```python
from build123d import *

# Parameters (mm, degrees)
SKETCH1_W           = 27.5
SKETCH1_H           = 40
BOSS_EXTRUDE1_DEPTH = 6.5
SKETCH2_W           = 17.25
SKETCH2_H           = 15.4
CUT_EXTRUDE1_DEPTH  = 1.15
SKETCH3_W           = 15.312161922
SKETCH3_H           = 2.25
CUT_EXTRUDE2_DEPTH  = 1.15


with BuildPart() as part:
    # Sketch1 → Boss-Extrude1 (new body)
    with BuildSketch(Plane.XY):
        Rectangle(SKETCH1_W, SKETCH1_H)
    extrude(amount=BOSS_EXTRUDE1_DEPTH)

    # Sketch2 → Cut-Extrude1 (cut)
    with BuildSketch(Plane(origin=(0, 0, 0), x_dir=(-1, 0, 0), z_dir=(0, 0, -1))):
        with Locations((-5.125, 1.9)):
            Rectangle(SKETCH2_W, SKETCH2_H)
    extrude(amount=-CUT_EXTRUDE1_DEPTH, mode=Mode.SUBTRACT)

    # Sketch3 → Cut-Extrude2 (cut)
    with BuildSketch(Plane(origin=(0, 0, 0), x_dir=(-1, 0, 0), z_dir=(0, 0, -1))):
        with Locations((0.219698945, -18.875)):
            Rectangle(SKETCH3_W, SKETCH3_H)
    extrude(amount=-CUT_EXTRUDE2_DEPTH, mode=Mode.SUBTRACT)


solid = part.part
```
Check sheet for the modelled part. Datum: model origin and axes. Units: mm. A direction names the side the tool comes from. Coordinates: 2 decimals unless noted, no trailing zeros. Write each loop counter-clockwise with the first axis right and the second up, starting at its lowest first coordinate (ties: lowest second). Pieces come first, ordered by that corner, then holes. Notation, with made-up numbers: M 1.5,26 L 60.5,26 A23 ccw 60.5,39 Z; hole C 81,16 d6. An arc over 180 degrees is marked long. Use one line per item in the form item = value.
Item 1: Sectioned sample at B-B, the plane z = 0.75. Record the cut outline in (x, y).
Answer below:
outline = M -13.75,-20 L -7.88,-20 L -7.88,-17.75 L 7.44,-17.75 L 7.44,-20 L 13.75,-20 L 13.75,-5.8 L -3.5,-5.8 L -3.5,9.6 L 13.75,9.6 L 13.75,20 L -13.75,20 Z
Item 2: Sectioned sample at A-A, the plane x = 6.25. Record the cut outline in (y, z), and give its area (3 significant figures).
Answer below:
outline = M -20,1.15 L -17.75,1.15 L -17.75,0 L -5.8,0 L -5.8,1.15 L 9.6,1.15 L 9.6,0 L 20,0 L 20,6.5 L -20,6.5 Z
area = 240 mm^2
Item 3: Release check for a two-part mould opening along Y. For faces 4 (the face through (0, 20, 3)), 5 (the face through (-13.75, 0, 3)), 6 (the face through (5.2, 9.6, 0.6)) record: pulls with the +Y half, pulls with the -Y half, needs draft (parallel to the pull), parting line crosses it, or undercut.
Answer below:
face_4 = pulls with the +Y half
face_5 = needs draft
face_6 = undercut
Item 4: Material ranges on L1, parallel to Y at x = 4.25, z = 0.5; L2, parallel to X at y = -4, z = 1; L3, parallel to Z at x = 1, y = -2, recorded low to high. Write a range as from..to.
Answer below:
L1 = -17.75..-5.8, 9.6..20
L2 = -13.75..-3.5
L3 = 1.15..6.5
Item 5: Sectioned sample at C-C, the plane y = -3. Record the cut outline in (x, z), and give its area (3 significant figures).
Answer below:
outline = M -13.75,0 L -3.5,0 L -3.5,1.15 L 13.75,1.15 L 13.75,6.5 L -13.75,6.5 Z
area = 159 mm^2
Item 6: Gauge pin test, flat ends, axial feed: pin 1 Ø0.7 at (x, y) = (-1, -19) entering from -Z; pin 2 Ø3 at (x, y) = (-5, -1) entering from -Z; pin 3 Ø0.6 at (x, z) = (4, 0.5) entering from -Y. Record the tip position at first contact, or that the pin passes through.
Answer below:
pin_1 = 1.15
pin_2 = 0
pin_3 = -17.75
Item 7: Set-up check for faces 1 (the face through (-0.1, -17.75, 0.6)), 2 (the face through (-3.5, 1.8, 0.6)), 3 (the face through (13.75, 0, 3)): record each of +Z, -Z, +X, -X, +Y, -Y from which the full face is reachable in a straight line by a thin tool's end or side.
Answer below:
face_1 = -Z, -Y
face_2 = -Z, +X
face_3 = +Z, -Z, +X, +Y, -Y
